from build123d import *

# Parameters (mm, degrees)
SKETCH2_R         = 10
EXTRUDE1_DEPTH    = 10
CIRPATTERN1_COUNT = 5
SKETCH3_W         = 4.5
SKETCH3_H         = 2.3
EXTRUDE2_DEPTH    = 16


with BuildPart() as part:
    # Sketch1 → Revolve1 (revolve)
    with BuildSketch(Plane.XY):
        with BuildLine():
            Line((-7.5, 7.5), (7.5, 7.5))
            Line((7.5, 7.5), (7.5, 17.5))
            Line((7.5, 17.5), (7, 17.5))
            ThreePointArc((7, 17.5), (5.585786438, 18.085786438), (5, 19.5))
            Line((5, 19.5), (5, 60))
            ThreePointArc((5, 60), (5.585786438, 61.414213562), (7, 62))
            Line((7, 62), (7.5, 62))
            Line((7.5, 62), (7.5, 70))
            Line((7.5, 70), (4.5, 70))
            Line((4.5, 70), (2.5, 62.5))
            Line((2.5, 62.5), (-2.5, 62.5))
            Line((-2.5, 62.5), (-4.5, 70))
            Line((-4.5, 70), (-7.5, 70))
            Line((-7.5, 70), (-7.5, 62))
            Line((-7.5, 62), (-7, 62))
            ThreePointArc((-7, 62), (-5.585786438, 61.414213562), (-5, 60))
            Line((-5, 60), (-5, 19.5))
            ThreePointArc((-5, 19.5), (-5.585786438, 18.085786438), (-7, 17.5))
            Line((-7, 17.5), (-7.5, 17.5))
            Line((-7.5, 17.5), (-7.5, 7.5))
        make_face()
    revolve(axis=Axis((25.864037296, 0, 0), (-1, 0, 0)))

    # Sketch2 → Extrude1 (cut)
    with BuildSketch(Plane(origin=(5, 0, 0), x_dir=(0, 0, -1), z_dir=(1, 0, 0))):
        with Locations((0, 39.75)):
            Circle(SKETCH2_R)
    extrude1 = extrude(amount=-EXTRUDE1_DEPTH, mode=Mode.SUBTRACT)

    # CirPattern1: Extrude1 ×5 about axis
    cirpattern1_axis = Axis((0, 0, 0), (1, 0, 0))
    for i in range(1, CIRPATTERN1_COUNT):
        add(extrude1.rotate(cirpattern1_axis, i * 360 / CIRPATTERN1_COUNT), mode=Mode.SUBTRACT)

    # Sketch3 → Extrude2 (cut, through all)
    with BuildSketch(Plane(origin=(7.5, 0, 0), x_dir=(0, 0, -1), z_dir=(1, 0, 0))):
        with Locations((0, -8.15)):
            Rectangle(SKETCH3_W, SKETCH3_H)
    extrude(amount=-EXTRUDE2_DEPTH, mode=Mode.SUBTRACT)


solid = part.part
Could you check a few things on this model? Use its own coordinates, in mm. A direction names the side the tool comes from. Give positions to 0.01 mm unless a question says otherwise; leave off trailing zeros. Write each loop counter-clockwise with the first axis right and the second up, starting at its lowest first coordinate (ties: lowest second). Pieces come first, ordered by that corner, then holes. Notation, with made-up numbers: (68.5, 14) -> (109.5, 14) arc R31 ccw to (109.5, 52) -> close; hole circle Ø1 at (7.25, 82.5). An arc over 180 degrees is marked (long way). Write each question's results on one line, items separated by ' | '. Start each with the question number.
Q1. Which directions (+Z, -Z, +X, -X, +Y, -Y) give clear straight access to the entire face, cutting with the end or side of a thin tool? Please do faces 1 (the face through (2.597, -13.628, 61.369)), 2 (the face through (7.246, -13.887, 10.648)), 3 (the face through (-5, -14, -14)).
Q2. I need wall thicknesses on probe 1 along Z at (x, y) = (7.3, 0); probe 2 along Y at (x, z) = (-7.35, 0); probe 3 along Y at (x, z) = (0.5, 0). Which ranges of each line are inside material? Lowest first, please.
Q3. We'd pull the mould along Y, two halves only. Please class faces 4 (the face through (-7.254, -13.887, 10.648)), 5 (the face through (7.5, 6, 62)), 6 (the face through (-2.625, -8.197, -62.433)): +Y half, -Y half, draft (parallel to the pull), parting line (faces both ways), or undercut.
Q4. Suppose I cut it at A-A, the plane x = 0. List the corners of the cut face in (y, z) for me.
Q5. Suppose I cut it at B-B, the plane z = 0. State how many separate pieces and enclosed holes the cut face has, and give its area (3 significant figures).
Q6. I'm going to push flat-ended pins straight in: pin 1 Ø0.6 at (x, y) = (1.5, -8.5) entering from +Z; pin 2 Ø4 at (y, z) = (6.5, 47.5) entering from -X; pin 3 Ø2 at (x, z) = (-5.5, 6.5) entering from +Y; pin 4 Ø3.5 at (x, z) = (3.5, -1) entering from +Y. Where does each tip first touch, or does it pass through?
Outcome:
1) face 1: none | face 2: +X | face 3: -X
2) probe 1: -70 to -62, -17.5 to -7.5, 7.5 to 17.5, 62 to 70 | probe 2: -70 to -62, -17.5 to -9.3, 7.5 to 17.5, 62 to 70 | probe 3: -62.5 to -9.3, 7.5 to 29.75, 49.75 to 62.5
3) face 4: undercut | face 5: draft | face 6: parting line
4) outline: circle Ø125 at (0, 0); hole circle Ø20 at (-32.16, -23.36); hole circle Ø20 at (-32.16, 23.36); hole (-9.3, -2.25) -> (-7.15, -2.25) arc R7.5 ccw (long way) to (-7.15, 2.25) -> (-9.3, 2.25) -> close; hole circle Ø20 at (12.28, -37.8); hole circle Ø20 at (12.28, 37.8); hole circle Ø20 at (39.75, 0)
5) separate pieces: 3 | enclosed holes: 0 | area: 1,100 mm2
6) pin 1: z = 61.96 | pin 2: x = -5 | pin 3: y = 69.78 | pin 4: y = 70
